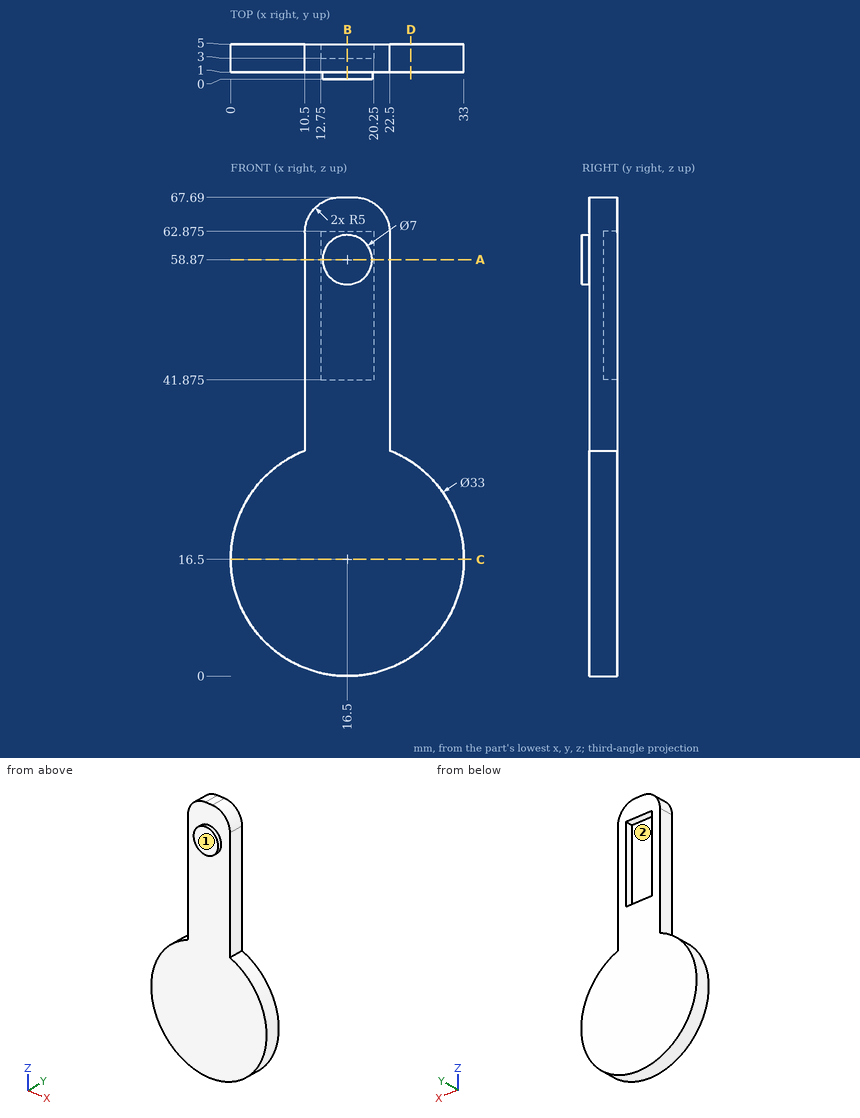
Geometry: see drawing. Coordinates: mm, zero at the bounding-box minimum. Give positions to 0.01 mm unless a question says otherwise; leave off trailing zeros. Loops run counter-clockwise (first coordinate to the right, second up) from the corner with the lowest first, then second, coordinate; pieces in that order, holes last. Notation, with made-up numbers: (-11.5, 19) - (22.5, 19) arc R20 ccw to (22.5, 31) - close; hole circle Ø5 at (13, 50.5). An arc over 180 degrees is marked (long way). One line per question, with ' | ' between items. Start each with the question number.
(1) Section query A-A on z = 58.87. Return loops of the section in (x, y), then the cut area to 3 significant figures.
(2) Ray query, line 1 (X direction, y = 4.3, z = 44); line 2 (Y direction, x = 24.5, z = 25); line 3 (X direction, y = 2.7, z = 53). Return the intervals inside material, ascending. Write a range as from..to.
(3) Section query C-C on z = 16.5. Return loops of the section in (x, y), then the cut area to 3 significant figures.
(4) Section query D-D on x = 25.5. Return loops of the section in (y, z), then the cut area to 3 significant figures.
(5) Pull-direction query (X, two-part tool) for the marked faces 1 and 2; classes: released by +X, released by -X, zero draft, split by the parting line, or undercut.
(6) Contact query for flat-ended pins moving along their axis: pin 1 (2 mm diameter, centred on y = 2.5, z = 33, fed in from +X); pin 2 (1.6 mm diameter, centred on y = 4, z = 54, fed in from -X); pin 3 (4 mm diameter, centred on x = 16, z = 52.5, fed in from +Y). Output: stop coordinate, or through.
(7) Section query B-B on x = 16.5. Return loops of the section in (y, z) (3 decimals).
The answers:
1) outline: (10.5, 1) - (13, 1) - (13, 0) - (20, 0) - (20, 1) - (22.5, 1) - (22.5, 5) - (20.25, 5) - (20.25, 3) - (12.75, 3) - (12.75, 5) - (10.5, 5) - close | area: 40.0 mm2
2) line 1: 10.5..12.75, 20.25..22.5 | line 2: 1..5 | line 3: 10.5..22.5
3) outline: (0, 1) - (33, 1) - (33, 5) - (0, 5) - close | area: 132 mm2
4) outline: (1, 2.67) - (5, 2.67) - (5, 30.33) - (1, 30.33) - close | area: 111 mm2
5) face 1: zero draft | face 2: undercut
6) pin 1: x = 22.5 | pin 2: x = 10.5 | pin 3: y = 3
7) outline: (0, 55.37) - (1, 55.37) - (1, 0) - (5, 0) - (5, 41.875) - (3, 41.875) - (3, 62.875) - (5, 62.875) - (5, 67.69) - (1, 67.69) - (1, 62.37) - (0, 62.37) - close
